Can you work these out from the drawing? Everything is in mm from the part's minimum corner. Give positions to 0.01 mm unless a question says otherwise; leave off trailing zeros. Loops run counter-clockwise (first coordinate to the right, second up) from the corner with the lowest first, then second, coordinate; pieces in that order, holes last. Notation, with made-up numbers: (-7, 65.5) -> (-3, 65.5) arc R28 ccw to (-3, 104.5) -> close; hole circle Ø3 at (64.25, 56.25). An arc over 180 degrees is marked (long way). Return JSON: item names as keys, results as strings. Group by question number.
Q1. Suppose I cut it at D-D, the plane x = 2.5. Please give me the cut outline in (y, z).
Q2. Suppose I cut it at A-A, the plane x = 25. Please give me the cut outline in (y, z).
Q3. Suppose I cut it at C-C, the plane y = 10. Please give me the cut outline in (x, z), and give its area (3 significant figures).
Q4. Suppose I cut it at B-B, the plane z = 2.45. Please give me the cut outline in (x, y).
Q5. Will these pins go through, and if not, where does the flat tip stop? pin 1 (3.5 mm diameter, centred on x = 10, y = 10, fed in from +Z); pin 2 (12 mm diameter, centred on x = 9, y = 19.5, fed in from -Z).
Q6. I need wall thicknesses on line 1 along Y through (x, z) = (10, 1.45); line 2 along Y through (x, z) = (25, 1.8); line 3 along X through (y, z) = (11.5, 2.4). Which ranges of each line are inside material? Lowest first, please. Write a range as [from, to].
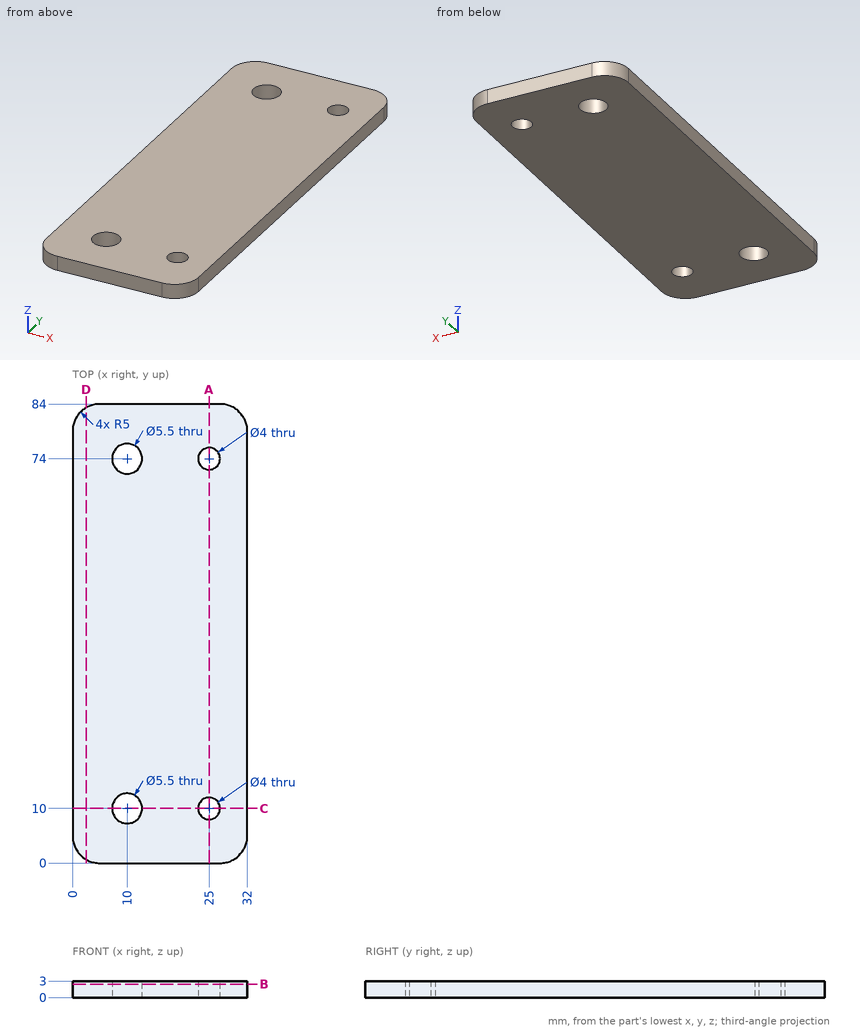
Ans:
{
 "1": {"outline": "(0.67, 0) -> (83.33, 0) -> (83.33, 3) -> (0.67, 3) -> close"},
 "2": {"outline": "(0, 0) -> (8, 0) -> (8, 3) -> (0, 3) -> close; (12, 0) -> (72, 0) -> (72, 3) -> (12, 3) -> close; (76, 0) -> (84, 0) -> (84, 3) -> (76, 3) -> close"},
 "3": {"outline": "(0, 0) -> (7.25, 0) -> (7.25, 3) -> (0, 3) -> close; (12.75, 0) -> (23, 0) -> (23, 3) -> (12.75, 3) -> close; (27, 0) -> (32, 0) -> (32, 3) -> (27, 3) -> close", "area": "67.5 mm^2"},
 "4": {"outline": "(0, 5) arc R5 ccw to (5, 0) -> (27, 0) arc R5 ccw to (32, 5) -> (32, 79) arc R5 ccw to (27, 84) -> (5, 84) arc R5 ccw to (0, 79) -> close; hole circle Ø5.5 at (10, 10); hole circle Ø5.5 at (10, 74); hole circle Ø4 at (25, 10); hole circle Ø4 at (25, 74)"},
 "5": {"pin 1": "passes through", "pin 2": "stops at z = 0"},
 "6": {"line 1": "y = [0, 7.25], [12.75, 71.25], [76.75, 84]", "line 2": "y = [0, 8], [12, 72], [76, 84]", "line 3": "x = [0, 7.7], [12.3, 23.68], [26.32, 32]"}
}
